CAD build for the part. Positions are in the model's coordinates, mm. A direction names the side the tool comes from. Coordinates: 2 decimals unless noted, no trailing zeros. Loops run counter-clockwise (first coordinate to the right, second up) from the corner with the lowest first, then second, coordinate; pieces in that order, holes last. Notation, with made-up numbers: (81.5, 30) -> (116.5, 30) arc R37 cw to (116.5, 69) -> close; hole circle Ø3 at (68, 88.5). An arc over 180 degrees is marked (long way). Answer as CSV lines item,"result". Start each with the question number.
```python
from build123d import *

# Parameters (mm, degrees)
SKETCH_1_R          = 2
EXTRUDE_1_DEPTH     = 8.75
SKETCH_2_R          = 2.1
EXTRUDE_2_DEPTH     = 1.2
CHAMFER_1_SIZE      = 0.2
SKETCH_3_W          = 0.8
SKETCH_3_H          = 4.5
CUT_EXTRUDE_1_DEPTH = 5.5


# Read off the part's stored shape, not the designer's step: 镜向1
with BuildPart() as part:
    # 草图1 → 凸台-拉伸1 (new body)
    with BuildSketch(Plane.XY):
        Circle(SKETCH_1_R)
    extrude(amount=EXTRUDE_1_DEPTH)

    # 草图2 → 凸台-拉伸2 (add)
    with BuildSketch(Plane.XY.offset(8.75)):
        Circle(SKETCH_2_R)
    extrude(amount=-EXTRUDE_2_DEPTH)

    # 倒角1
    chamfer_1_edges = [part.edges().sort_by_distance(p)[0] for p in [
        (-2.1, 0, 8.75),
    ]]
    chamfer(chamfer_1_edges, length=CHAMFER_1_SIZE)

    # 草图3 → 切除-拉伸1 (cut)
    with BuildSketch(Plane.XY.offset(8.75)):
        Rectangle(SKETCH_3_W, SKETCH_3_H)
    extrude(amount=-CUT_EXTRUDE_1_DEPTH, mode=Mode.SUBTRACT)

    # 镜向1: part across plane


with BuildPart() as part_1:
    add(part.part)
    add(part.part.mirror(Plane.XY))


solid = part_1.part
```
Q1. Saw through at A-A (y = 0). List the corners of the cut face in (x, z).
Q2. Pin check, flat tip, straight feed: pin 1 Ø1.5 at (y, z) = (1, -5) entering from -X. Stop position of the tip, or through.
Q3. Saw through at D-D (z = 7). List the corners of the cut face in (x, y).
Q4. Probe probe 1 along X at (y, z) = (-1.65, 4.25); probe 2 along Z at (x, y) = (-0.25, 0.5); probe 3 along X at (y, z) = (0.7, 5.25). List the from-to ranges inside material, lowest first. Write a range as from..to.
Q5. Two-plate mould, pull along X, no slides. Class faces 1 (the flat face through (-1, 0, -8.75)), 2 (the flat face through (0.4, 0, 6)), 3 (the flat face through (0, 0, 3.25)), 4 (the cylindrical face through (-2.1, 0, 8.1)): pulls with the +X half, pulls with the -X half, needs draft (parallel to the pull), parting line crosses it, or undercut.
Q6. Which spindle directions (+Z, -Z, +X, -X, +Y, -Y) get a long thin tool onto all of the face, cutting with end or side? Do faces 5 (the flat face through (1, 0, 8.75)), 6 (the flat face through (-0.4, 0, 6)), 7 (the flat face through (0.4, 0, -6)). Say none if no direction does.
Q7. Saw through at B-B (x = 0). List the corners of the cut face in (y, z).
Q8. Saw through at C-C (z = 2.5). List the corners of the cut face in (x, y).
Ans:
1,outline,"(-2.1, -8.55) -> (-1.9, -8.75) -> (-0.4, -8.75) -> (-0.4, -3.25) -> (0.4, -3.25) -> (0.4, -8.75) -> (1.9, -8.75) -> (2.1, -8.55) -> (2.1, -7.55) -> (2, -7.55) -> (2, 7.55) -> (2.1, 7.55) -> (2.1, 8.55) -> (1.9, 8.75) -> (0.4, 8.75) -> (0.4, 3.25) -> (-0.4, 3.25) -> (-0.4, 8.75) -> (-1.9, 8.75) -> (-2.1, 8.55) -> (-2.1, 7.55) -> (-2, 7.55) -> (-2, -7.55) -> (-2.1, -7.55) -> close"
2,pin 1,"stops at x = -1.98"
3,outline,"(-0.4, -1.96) -> (-0.4, 1.96) arc R2 ccw to start; (0.4, -1.96) arc R2 ccw to (0.4, 1.96) -> close"
4,probe 1,"x = -1.13..-0.4, 0.4..1.13"
4,probe 2,"z = -3.25..3.25"
4,probe 3,"x = -1.87..-0.4, 0.4..1.87"
5,face 1,"needs draft"
5,face 2,"undercut"
5,face 3,"undercut"
5,face 4,"pulls with the -X half"
6,face 5,"+Z, +X, -X, +Y, -Y"
6,face 6,"+Z, +Y, -Y"
6,face 7,"-Z, +Y, -Y"
7,outline,"(-2, -3.25) -> (2, -3.25) -> (2, 3.25) -> (-2, 3.25) -> close"
8,outline,"circle Ø4 at (0, 0)"
